Source: CAD feature listing. Evaluate the final solid. Frame: model axes, mm. A direction names the side the tool comes from. Give positions to 0.01 mm unless a question says otherwise; leave off trailing zeros. Loops run counter-clockwise (first coordinate to the right, second up) from the corner with the lowest first, then second, coordinate; pieces in that order, holes last. Notation, with made-up numbers: (22, -2) -> (45, -2) arc R24 ccw to (45, 33) -> close; hole circle Ø6 at (17.5, 58). An arc over 180 degrees is marked (long way). Put each result on its own line as item: value.
```python
from build123d import *

# Parameters (mm, degrees)
SKETCH2_R           = 2.8
BOSS_EXTRUDE1_DEPTH = 5
BOSS_EXTRUDE2_DEPTH = 5
SKETCH4_R           = 3.5
CUT_EXTRUDE1_DEPTH  = 10


with BuildPart() as part:
    # Sketch2 → Boss-Extrude1 (new body)
    with BuildSketch(Plane.XY):
        with BuildLine():
            Line((0, 0), (15, 0))
            Line((15, 0), (15, 20))
            ThreePointArc((15, 20), (7.5, 27.5), (0, 20))
            Line((0, 20), (0, 0))
        make_face()
        with Locations((7.5, 5)):
            Circle(SKETCH2_R, mode=Mode.SUBTRACT)
    extrude(amount=BOSS_EXTRUDE1_DEPTH)

    # Sketch3 → Boss-Extrude2 (add)
    with BuildSketch(Plane(origin=(0, 0, 0), x_dir=(-1, 0, 0), z_dir=(0, 0, -1))):
        with BuildLine():
            Line((-15, 20), (-15, 15))
            Line((-15, 15), (0, 15))
            Line((0, 15), (0, 20))
            ThreePointArc((0, 20), (-7.5, 27.5), (-15, 20))
        make_face()
    extrude(amount=BOSS_EXTRUDE2_DEPTH)

    # Sketch4 → Cut-Extrude1 (cut)
    with BuildSketch(Plane(origin=(5.915063509, 0, 10.245190528), x_dir=(0, 1, 0), z_dir=(0.5, 0, 0.866025404))):
        with Locations((20, -5.490381057)):
            Circle(SKETCH4_R)
    extrude(amount=-CUT_EXTRUDE1_DEPTH, mode=Mode.SUBTRACT)


solid = part.part
```
(1) Reachability of faces 4 (the flat face through (7, 14, 5)), 5 (the flat face through (7, 9, 0)) from +Z, -Z, +X, -X, +Y, -Y: full face, straight path, thin tool, end or side. Return the list, or none.
Calculated:
face 4: +Z, +X, -X, +Y, -Y
face 5: -Z, +X, -X, -Y
(2) First-contact query: P1, Ø1.5, axis at x = 10.5, y = 19.5, coming from the +Z side; P2, Ø4.5, axis at x = 7.5, y = 5, coming from the -Z side; P3, Ø1, axis at x = 10.5, z = -1.5, coming from the -Y side. Flat tips, straight axial feed; report the tip coordinate or a pass-through.
Calculated:
P1: stops at z = 1.6
P2: passes through
P3: stops at y = 15
(3) Section C-C on z = 3. Give the number of separate pieces and of enclosed holes in the cut face, then the cut area to 3 significant figures.
Calculated:
separate pieces: 1
enclosed holes: 2
area: 319 mm²
(4) Line query: probe 1 along Y at (x, z) = (7.5, 2.25); probe 2 along Z at (x, y) = (8.25, 9.5); probe 3 along Y at (x, z) = (5.75, 4). Output: solid intervals per line, ascending. Write a range as from..to.
Calculated:
probe 1: y = 0..2.2, 7.8..16.5, 23.5..27.5
probe 2: z = 0..5
probe 3: y = 0..2.81, 7.19..17.56, 22.44..27.29
(5) Draft query along X for faces 1 (the flat face through (8, 15, -2)), 2 (the flat face through (5.627, 19.951, -1.136)), 3 (the cylindrical face through (7.34, 27.5, 0.07)). Return one class per face: released by +X, released by -X, zero draft, split by the parting line, or undercut.
Calculated:
face 1: zero draft
face 2: undercut
face 3: split by the parting line
(6) Section A-A on y = 5. Return loops of the section in (x, z), then the cut area to 3 significant figures.
Calculated:
outline: (0, 0) -> (4.7, 0) -> (4.7, 5) -> (0, 5) -> close; (10.3, 0) -> (15, 0) -> (15, 5) -> (10.3, 5) -> close
area: 47.0 mm²
(7) Section D-D on y = 12.75. Return loops of the section in (x, z).
Calculated:
outline: (0, 0) -> (15, 0) -> (15, 5) -> (0, 5) -> close
(8) Section B-B on y = 21. Return loops of the section in (x, z), then the cut area to 3 significant figures.
Calculated:
outline: (0.07, -5) -> (14.93, -5) -> (14.93, 5) -> (13.1, 5) -> (8.57, -2.84) -> (2.77, 0.52) -> (5.35, 5) -> (0.07, 5) -> close
area: 101 mm²
